The figure shows three views and two pictorial views of one solid part (mm, origin at its lowest corner). Answer the questions. A direction names the side the tool comes from. Coordinates: 2 decimals unless noted, no trailing zeros. Write each loop counter-clockwise with the first axis right and the second up, starting at its lowest first coordinate (ties: lowest second). Pieces come first, ordered by that corner, then holes. Notation, with made-up numbers: M 0.25,6 L 59.25,6 A18 ccw 59.25,16 Z; hole C -26.75,4 d7. An arc over 180 degrees is marked long. Write item = value, one per line.
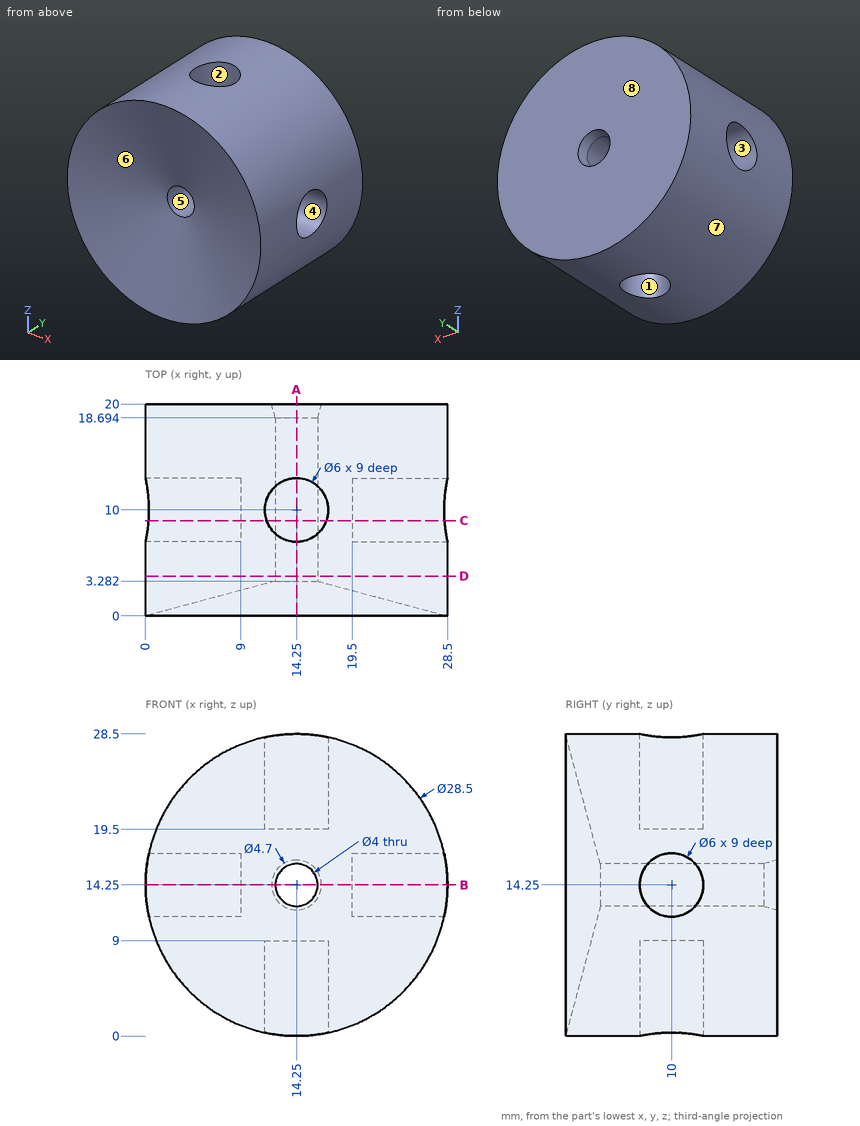
Item 1: Find section D-D (y = 3.75). Determine the outline of the cut face in (x, z), and give its area (3 significant figures).
Worked answers:
outline = C 14.25,14.25 d28.5; hole C 14.25,14.25 d4
area = 625 mm²
Item 2: Find section C-C (y = 9). Determine the outline of the cut face in (x, z).
Worked answers:
outline = M 0.28,11.42 A14.25 ccw 11.42,0.28 L 11.42,9 L 17.08,9 L 17.08,0.28 A14.25 ccw 28.22,11.42 L 19.5,11.42 L 19.5,17.08 L 28.22,17.08 A14.25 ccw 17.08,28.22 L 17.08,19.5 L 11.42,19.5 L 11.42,28.22 A14.25 ccw 0.28,17.08 L 9,17.08 L 9,11.42 Z; hole C 14.25,14.25 d4
Item 3: Find section A-A (x = 14.25). Determine the outline of the cut face in (y, z).
Worked answers:
outline = M 0,0 L 7,0 L 7,9 L 13,9 L 13,0 L 20,0 L 20,11.9 L 18.69,12.25 L 3.28,12.25 Z; M 0,28.5 L 3.28,16.25 L 18.69,16.25 L 20,16.6 L 20,28.5 L 13,28.5 L 13,19.5 L 7,19.5 L 7,28.5 Z
Item 4: Find section B-B (z = 14.25). Determine the outline of the cut face in (x, y), and give its area (3 significant figures).
Worked answers:
outline = M 0,0 L 12.25,3.28 L 12.25,18.69 L 11.9,20 L 0,20 L 0,13 L 9,13 L 9,7 L 0,7 Z; M 16.25,3.28 L 28.5,0 L 28.5,7 L 19.5,7 L 19.5,13 L 28.5,13 L 28.5,20 L 16.6,20 L 16.25,18.69 Z
area = 341 mm²
Item 5: For a pull along X with two mould halves and no side action, classify the marked faces 5, 6, 7 and 8 as released by +X, released by -X, zero draft, split by the parting line, or undercut.
Worked answers:
face_5 = undercut
face_6 = undercut
face_7 = split by the parting line
face_8 = zero draft
Item 6: Which of the six approach directions +Z, -Z, +X, -X, +Y, -Y give full straight-line access (tool end or side, diameter ignored) to the marked faces 1, 2, 3 and 4?
Worked answers:
face_1 = -Z
face_2 = +Z
face_3 = -X
face_4 = +X
Item 7: Consider line 1 along X through (y, z) = (9, 14.25); line 2 along Y through (x, z) = (13, 1.75); line 3 along Z through (x, y) = (27, 8) (1 decimal). Determine where each line is inside the solid, lowest interval first. Write a range as from..to.
Worked answers:
line_1 = 9..12.25, 16.25..19.5
line_2 = 0.45..7.27, 12.73..20
line_3 = 7.9..12, 16.5..20.6
Item 8: Flat-ended cylindrical pins translate along their axes: pin 1 (6.5 mm diameter, centred on y = 8.5, z = 14.5, fed in from -X); pin 2 (6 mm diameter, centred on x = 13, z = 4, fed in from -Y); pin 3 (10 mm diameter, centred on x = 4.5, y = 17, fed in from +Z) (1 decimal); pin 4 (3.5 mm diameter, centred on x = 14.25, y = 10, fed in from +Z). Find the tip coordinate at first contact, or state that the pin passes through.
Worked answers:
pin_1 = 0
pin_2 = 0.25
pin_3 = 27.7
pin_4 = 19.5
